```python
from build123d import *

# Parameters (mm, degrees)
BOSS_EXTRUDE1_DEPTH = 2.54
F_3DSKETCH1_R       = 2.75
BOSS_EXTRUDE3_DEPTH = 2


with BuildPart() as part:
    # Sketch1 → Boss-Extrude1 (new body)
    with BuildSketch(Plane(origin=(0, 0, 0), x_dir=(1, 0, 0), z_dir=(0, 1, 0))):
        Polygon((-24.263943822, 4.856129722), (-24.263943822, -1.143870278), (-22.263943822, -1.143870278), (-22.263943822, 2.856129722), (-14.821743822, 2.856129722), (-14.821743822, 4.856129722), align=None)
    extrude(amount=BOSS_EXTRUDE1_DEPTH)

    # 3DSketch1 → Boss-Extrude3 (add)
    with BuildSketch(Plane(origin=(-14.821743822, 5.174700089, 5.887638741), x_dir=(0, -0.5879624138152767, -0.808888249352476), z_dir=(1, 0, 0))):
        Polygon((0, 0), (4.591633779, -6.316932039), (13.282141842, 0), (8.690508063, 6.316932039), align=None)
        with Locations(Location((4.966765889, -1.217014129, 0), (0, 0, 36.012547839))):
            Circle(F_3DSKETCH1_R, mode=Mode.SUBTRACT)
    extrude(amount=BOSS_EXTRUDE3_DEPTH)


solid = part.part
```
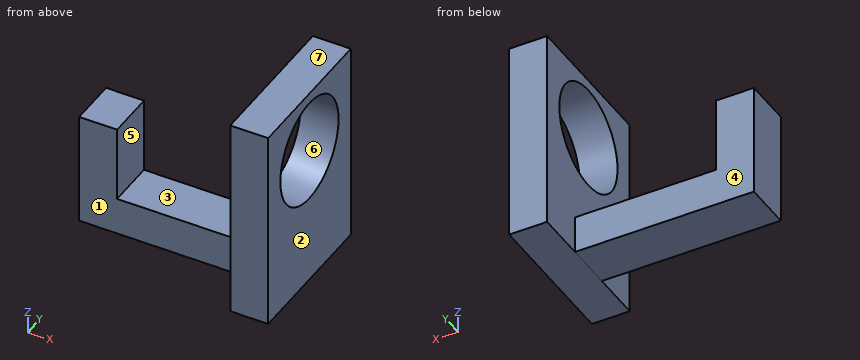
Read the model definition and answer for the solid it produces. Units are mm, in the model's axes. Face numbers are marked on the shaded views. A direction names the side the tool comes from. Round coordinates to 2 decimals unless told otherwise and drop trailing zeros. Write each loop counter-clockwise with the first axis right and the second up, starting at its lowest first coordinate (ties: lowest second). Pieces come first, ordered by that corner, then holes. Notation, with made-up numbers: (68.5, -3.5) - (85.5, -3.5) arc R10 cw to (85.5, 14.5) - close; hole circle Ø3 at (10, 56). An arc over 180 degrees is marked (long way). One line per item, written item: value.
Q1. Find section A-A (y = 1.27). Determine the outline of the cut face in (x, z).
The answers:
outline: (-24.26, -4.86) - (-12.82, -4.86) - (-12.82, -0.16) - (-14.82, -0.16) - (-14.82, -2.86) - (-22.26, -2.86) - (-22.26, 1.14) - (-24.26, 1.14) - close; (-14.82, 5.34) - (-12.82, 5.34) - (-12.82, 5.89) - (-14.82, 5.89) - close
Q2. Which of the six approach directions +Z, -Z, +X, -X, +Y, -Y give full straight-line access (tool end or side, diameter ignored) to the marked faces 1, 2, 3 and 4?
The answers:
face 1: +Z, -Z, -X, -Y
face 2: +Z, -Z, +X, +Y, -Y
face 3: +Z, +Y, -Y
face 4: +Z, -Z, -X, +Y
Q3. Straight lines are drawn through the part: line 1 (Z direction, x = -13.25, y = 1.27); line 2 (X direction, y = 0.75, z = -0.5); line 3 (X direction, y = 4.25, z = 3.5). For each, find the intervals that lie inside material, in ascending order. Write a range as from..to.
The answers:
line 1: z = -4.86..-0.16, 5.34..5.89
line 2: x = -24.26..-22.26, -14.82..-12.82
line 3: x = -14.82..-12.82
Q4. For a pull along Z with two mould halves and no side action, classify the marked faces 5, 6 and 7 as pulls with the +Z half, pulls with the -Z half, needs draft (parallel to the pull), parting line crosses it, or undercut.
The answers:
face 5: needs draft
face 6: undercut
face 7: pulls with the +Z half
Q5. Each of these flat-tipped pins is pushed along its axis until it touches: P1, Ø5, axis at x = -20, z = -1.5, coming from the +Y side; P2, Ø1, axis at x = -23, y = 1.5, coming from the +Z side; P3, Ø1, axis at y = 4, z = 0, coming from the -X side; P4, Ø3, axis at x = -18, z = 4.5, coming from the +Y side. Where does it stop, or does it pass through?
The answers:
P1: stops at y = 2.54
P2: stops at z = 1.14
P3: stops at x = -14.82
P4: passes through
Q6. Find section B-B (z = 1). Determine the outline of the cut face in (x, y).
The answers:
outline: (-24.26, 0) - (-22.26, 0) - (-22.26, 2.54) - (-24.26, 2.54) - close; (-14.82, -2.63) - (-12.82, -2.63) - (-12.82, -0.98) - (-14.82, -0.98) - close; (-14.82, 3.52) - (-12.82, 3.52) - (-12.82, 5.17) - (-14.82, 5.17) - close
Q7. Find section C-C (x = -22.5). Determine the outline of the cut face in (y, z).
The answers:
outline: (0, -4.86) - (2.54, -4.86) - (2.54, 1.14) - (0, 1.14) - close
Q8. Find section D-D (y = 3). Determine the outline of the cut face in (x, z).
The answers:
outline: (-14.82, -4.86) - (-12.82, -4.86) - (-12.82, 0.45) - (-14.82, 0.45) - close; (-14.82, 4.72) - (-12.82, 4.72) - (-12.82, 5.89) - (-14.82, 5.89) - close
